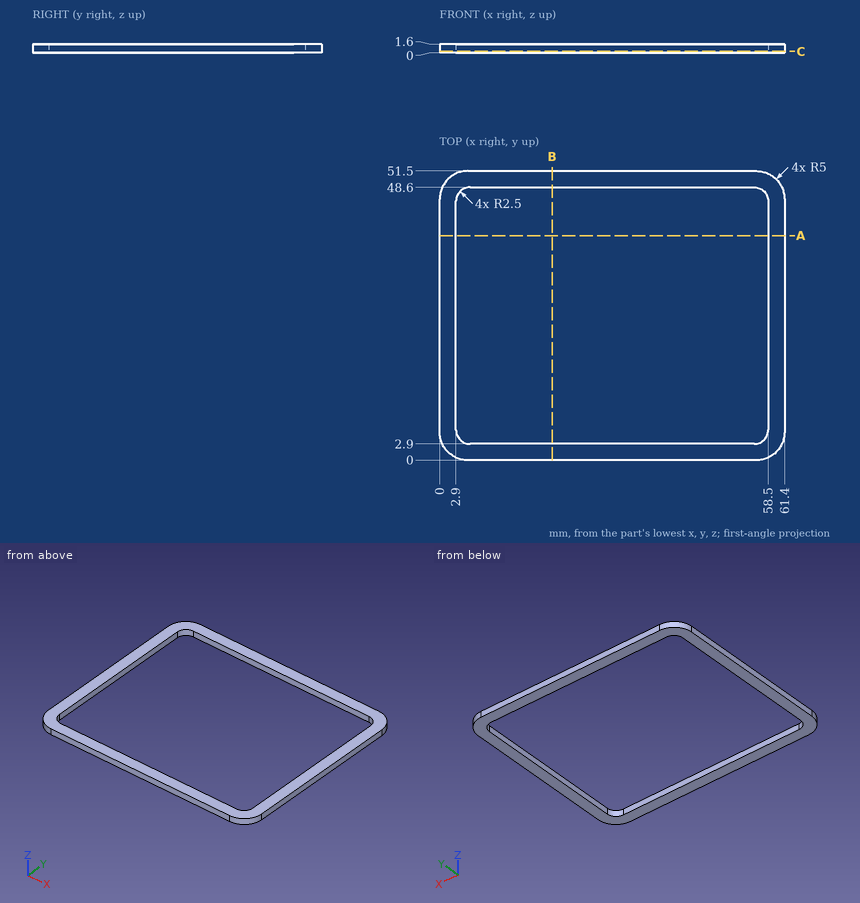
Could you check a few things on this drawing? It's one solid part, dimensions in mm from its lowest x, y, z. Give positions to 0.01 mm unless a question says otherwise; leave off trailing zeros. Order: outer loops, then holes, each group sorted by start corner. A loop starts at its lowest first (then second) coordinate and runs counter-clockwise, first axis right, second up. Notation, with made-up numbers: (29, 41.5) -> (44, 41.5) arc R11 cw to (44, 58.5) -> close; hole circle Ø2 at (13.5, -17.75). An arc over 180 degrees is marked (long way). Use CSV: the item, a comma, the result in double quotes. Start each with the question number.
Item 1: Suppose I cut it at A-A (y = 40). List the corners of the cut face in (x, z) for me, and give its area (3 significant figures).
Item 2: If I drill on probe 1 along X at (y, z) = (43.5, 0.7); probe 2 along Y at (x, z) = (43, 0.6), over which ranges is the centre line in solid material (lowest first)? Write a range as [from, to].
Item 3: Suppose I cut it at B-B (x = 20). List the corners of the cut face in (y, z) for me, and give its area (3 significant figures).
Item 4: I'm going to push a flat-ended pin straight in: P1, Ø12, axis at x = 39, y = 5.5, coming from the +Z side. Where does the tip first touch, or does it pass through?
Item 5: Suppose I cut it at C-C (z = 0.3). List the corners of the cut face in (x, y) for me, and give its area (3 significant figures).
Answer block:
1,outline,"(0, 0) -> (2.9, 0) -> (2.9, 1.6) -> (0, 1.6) -> close; (58.5, 0) -> (61.4, 0) -> (61.4, 1.6) -> (58.5, 1.6) -> close"
1,area,"9.28 mm^2"
2,probe 1,"x = [0, 2.9], [58.5, 61.4]"
2,probe 2,"y = [0, 2.9], [48.6, 51.5]"
3,outline,"(0, 0) -> (2.9, 0) -> (2.9, 1.6) -> (0, 1.6) -> close; (48.6, 0) -> (51.5, 0) -> (51.5, 1.6) -> (48.6, 1.6) -> close"
3,area,"9.28 mm^2"
4,P1,"stops at z = 1.6"
5,outline,"(0, 5) arc R5 ccw to (5, 0) -> (56.4, 0) arc R5 ccw to (61.4, 5) -> (61.4, 46.5) arc R5 ccw to (56.4, 51.5) -> (5, 51.5) arc R5 ccw to (0, 46.5) -> close; hole (2.9, 5.4) arc R2.5 ccw to (5.4, 2.9) -> (56, 2.9) arc R2.5 ccw to (58.5, 5.4) -> (58.5, 46.1) arc R2.5 ccw to (56, 48.6) -> (5.4, 48.6) arc R2.5 ccw to (2.9, 46.1) -> close"
5,area,"605 mm^2"
